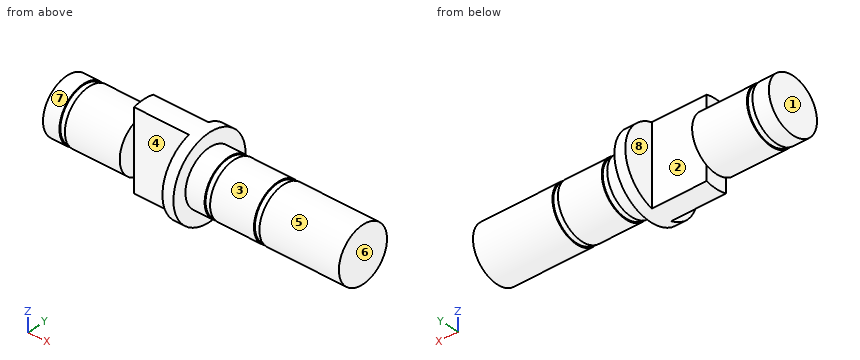
```python
from build123d import *

# Parameters (mm, degrees)
CUT_EXTRUDE8_DEPTH = 10


with BuildPart() as part:
    # Sketch3 → Revolve1 (revolve)
    with BuildSketch(Plane(origin=(0, 0, 0), x_dir=(1, 0, 0), z_dir=(0, 1, 0)), mode=Mode.PRIVATE) as revolve1_sk:
        Polygon((0, 0), (54, 0), (54, 4.99), (39.5, 4.99), (39.5, 4.79), (38.5, 4.79), (38.5, 4.99), (30.5, 4.99), (30.5, 4.79), (29.5, 4.79), (29.5, 4.99), (26, 4.99), (26, 7.49), (14, 7.49), (14, 4.99), (4, 4.99), (4, 4.79), (3, 4.79), (3, 4.99), (0, 4.99), align=None)
    revolve(revolve1_sk.sketch.rotate(Axis((0, 0, 0), (1, 0, 0)), 180), axis=Axis((0, 0, 0), (1, 0, 0)))

    # Sketch10 → Cut-Extrude8 (cut)
    with BuildSketch(Plane.ZY.offset(-14)):
        with BuildLine():
            Line((7.228416147, 2), (-7.228416147, 2))
            ThreePointArc((-7.228416147, 2), (0, 7.5), (7.228416147, 2))
        make_face()
        with BuildLine():
            Line((7.228416147, -2), (-7.228416147, -2))
            ThreePointArc((-7.228416147, -2), (0, -7.5), (7.228416147, -2))
        make_face()
    extrude(amount=-CUT_EXTRUDE8_DEPTH, mode=Mode.SUBTRACT)


solid = part.part
```
The listing builds one solid part. Answer for the finished solid, in the listing's coordinates (mm). Face numbers are marked on the shaded views. A direction names the side the tool comes from. Coordinates: 2 decimals unless noted, no trailing zeros. Order: outer loops, then holes, each group sorted by start corner. A loop starts at its lowest first (then second) coordinate and runs counter-clockwise, first axis right, second up. Notation, with made-up numbers: M -32,43 L 12,43 A11 ccw 12,60 Z; hole C 26.5,75.5 d9. An arc over 180 degrees is marked long. Answer as a JSON object with one key per item and string values. Group by question number.
1. Section C-C on x = 47 is taken. Write down the section's boundary in (y, z), then the cut area to 3 significant figures.
2. A tool of negligible diameter and unlimited length cuts with its end or side. For the marked faces 4, 5, 6, 7 and 8, from which of +Z, -Z, +X, -X, +Y, -Y can it reach the whole face along a straight path? Write none if from no direction.
3. Section B-B on y = -5.75 is taken. Write down the section's boundary in (x, z).
4. Section A-A on x = 18.5 is taken. Write down the section's boundary in (y, z).
5. Straight lines are drawn through the part: line 1 (X direction, y = 3.25, z = -3); line 2 (X direction, y = 6.25, z = -0.5); line 3 (Y direction, x = 18, z = 6). For each, find the intervals that lie inside material, in ascending order.
6. Determine the mould class of the marked faces 1, 2 and 3 for opening direction X: released by +X, released by -X, zero draft, split by the parting line, or undercut.
7. Flat-ended cylindrical pins translate along their axes: P1, Ø1, axis at x = 15.5, z = -2, coming from the +Y side; P2, Ø2, axis at x = 37, z = -1.5, coming from the +Y side; P3, Ø1, axis at x = 33, y = 5, coming from the +Z side. Find the tip coordinate at first contact, or state that the pin passes through.
Values follow:
{
 "1": {"outline": "C 0,0 d9.98", "area": "78.2 mm2"},
 "2": {"face 4": "+Z, -Z, -Y", "face 5": "+X", "face 6": "+Z, -Z, +X, +Y, -Y", "face 7": "-X", "face 8": "+Z, -Z, +Y"},
 "3": {"outline": "M 24,-4.8 L 26,-4.8 L 26,4.8 L 24,4.8 Z"},
 "4": {"outline": "M -2,-7.22 A7.49 ccw 2,-7.22 L 2,7.22 A7.49 ccw -2,7.22 Z"},
 "5": {"line 1": "0 to 14, 24 to 54", "line 2": "24 to 26", "line 3": "-2 to 2"},
 "6": {"face 1": "released by -X", "face 2": "undercut", "face 3": "zero draft"},
 "7": {"P1": "y = 2", "P2": "y = 4.96", "P3": "z = 2.16"}
}
